For this review, take the finished solid that the model builds, in its own axes (mm). A direction names the side the tool comes from. Coordinates: 2 decimals unless noted, no trailing zeros. Order: outer loops, then holes, each group sorted by start corner. A loop starts at its lowest first (then second) coordinate and runs counter-clockwise, first axis right, second up. Notation, with made-up numbers: (-19.5, -23) -> (2.5, -23) arc R33 cw to (2.5, 16) -> close; hole circle Ø1 at (31, -28). An arc over 180 degrees is marked (long way). Write item = value, one per line. Start each with the question number.
1) Wall thickness on probe 1 along X at (y, z) = (34, 3); probe 2 along Y at (x, z) = (32.5, -0.75); probe 3 along X at (y, z) = (17, -5.75): over which ranges is each line inside the solid? List them lowest first. Write a range as [from, to].
2) Consider section D-D on x = 22. Give the boundary of the cut face in (y, z), and give its area (3 significant figures).
3) Insertion check: pin 1 Ø5 at (x, z) = (63, 6) entering from -Y. The pin has a flat end and moves straight along its axis. Give the tip position at first contact, or say it passes through.
4) Consider section C-C on x = 61.5. Give the boundary of the cut face in (y, z), and give its area (3 significant figures).
5) Consider section B-B on z = -7.75. Give the boundary of the cut face in (x, y), and give its area (3 significant figures).
6) Consider section A-A on x = 35. Give the boundary of the cut face in (y, z), and give its area (3 significant figures).
7) Draft analysis for pull direction Y (two halves, no side actions). For faces 1 (the face through (45, 60, 0)), 2 (the face through (35, 35, 0)), 3 (the face through (65, 20, 0)), 4 (the face through (45, 35, 15)), state which applies: +Y half, -Y half, draft (parallel to the pull), parting line (faces both ways), or undercut.
8) Machinability: for faces 5 (the face through (80, 30, 0)), 6 (the face through (70, 15, 0)), 7 (the face through (45, 30, 0)), which of the approach directions +Z, -Z, +X, -X, +Y, -Y give a long, thin tool a straight path to every point of the face, cutting with its end or side? Answer none if there is none.
from build123d import *

# Parameters (mm, degrees)
SKETCH2_R           = 5
BOSS_EXTRUDE2_DEPTH = 15


with BuildPart() as part:
    # Sketch2 → Boss-Extrude2 (new, symmetric)
    with BuildSketch(Plane.XY):
        Polygon((10, 10), (10, 50), (20, 60), (70, 60), (80, 50), (80, 10), (70, 10), (70, 20), (60, 20), (60, 10), (30, 10), (30, 20), (20, 20), (20, 10), align=None)
        with Locations((20, 50)):
            Circle(SKETCH2_R, mode=Mode.SUBTRACT)
        with Locations(Location((70, 50, 0), (0, 0, 180))):
            Circle(SKETCH2_R, mode=Mode.SUBTRACT)
        Polygon((50, 30), (40, 30), (40, 35), (30, 35), (30, 25), (60, 25), (60, 35), (50, 35), align=None, mode=Mode.SUBTRACT)
    extrude(amount=BOSS_EXTRUDE2_DEPTH, both=True)


solid = part.part
Answer sheet:
q1.probe_1 = [10, 30], [40, 50], [60, 80]
q1.probe_2 = [10, 25], [35, 60]
q1.probe_3 = [10, 20], [30, 60], [70, 80]
q2.outline = (20, -15) -> (45.42, -15) -> (45.42, 15) -> (20, 15) -> close; (54.58, -15) -> (60, -15) -> (60, 15) -> (54.58, 15) -> close
q2.area = 925 mm2
q3.pin_1 = 20
q4.outline = (20, -15) -> (60, -15) -> (60, 15) -> (20, 15) -> close
q4.area = 1,200 mm2
q5.outline = (10, 10) -> (20, 10) -> (20, 20) -> (30, 20) -> (30, 10) -> (60, 10) -> (60, 20) -> (70, 20) -> (70, 10) -> (80, 10) -> (80, 50) -> (70, 60) -> (20, 60) -> (10, 50) -> close; hole circle Ø10 at (20, 50); hole (30, 25) -> (60, 25) -> (60, 35) -> (50, 35) -> (50, 30) -> (40, 30) -> (40, 35) -> (30, 35) -> close; hole circle Ø10 at (70, 50)
q5.area = 2,790 mm2
q6.outline = (10, -15) -> (25, -15) -> (25, 15) -> (10, 15) -> close; (35, -15) -> (60, -15) -> (60, 15) -> (35, 15) -> close
q6.area = 1,200 mm2
q7.face_1 = +Y half
q7.face_2 = undercut
q7.face_3 = -Y half
q7.face_4 = draft
q8.face_5 = +Z, -Z, +X, +Y, -Y
q8.face_6 = +Z, -Z, -Y
q8.face_7 = +Z, -Z
